Geometry check sheet. Reference: the model listing, model coordinates, mm. A direction names the side the tool comes from. Give positions to 0.01 mm unless a question says otherwise; leave off trailing zeros. Loops run counter-clockwise (first coordinate to the right, second up) from the corner with the lowest first, then second, coordinate; pieces in that order, holes last. Notation, with made-up numbers: (47, 67) -> (92, 67) arc R25 cw to (92, 93) -> close; hole circle Ø9 at (-3.75, 34.25). An arc over 180 degrees is marked (long way). Write item = value, one per line. Start each with the question number.
```python
from build123d import *

# Parameters (mm, degrees)
F0_R     = 4.35
F1_DEPTH = 15
F0_R_2   = 7
F2_DEPTH = 2
F3_D     = 5.5


with BuildPart() as f1:
    # F0 (on Top) → F1 (new body)
    with BuildSketch(Plane.XY):
        Circle(F0_R)
    extrude(amount=F1_DEPTH)

    # F0 (on Top) → F2 (join)
    with BuildSketch(Plane.XY):
        Circle(F0_R_2)
        Circle(F0_R, mode=Mode.SUBTRACT)
    extrude(amount=F2_DEPTH)

    # F3 (through all)
    with Locations(Plane(origin=(0, 0, 0), x_dir=(1, 0, 0), z_dir=(0, 0, -1))):
        with Locations((0, 0)):
            Hole(F3_D / 2)


solid = f1.part
```
1) Section check C-C (z = 6.75). Enter the section's corners in (x, y).
2) Section check D-D (x = 4). Enter the section's corners in (y, z), plus the area to 3 significant figures.
3) Draft check along X on faces 1 (the flat face through (0, -3, 0)), 2 (the cylindrical face through (6.466, -2.681, 0.986)), 3 (the cylindrical face through (0.596, 2.685, 7.605)). Enter one of: released by +X, released by -X, zero draft, split by the parting line, or undercut.
4) Section check A-A (x = 0). Enter the section's corners in (y, z), plus the area to 3 significant figures.
5) Thickness scan on line 1 (Y direction, x = 0, z = 5); line 2 (Z direction, x = -2.5, y = -4.75); line 3 (X direction, y = 0.5, z = 12). Record the ranges inside material, lowest first.
6) Tool access check on faces 4 (the flat face through (0, -3, 15)), 5 (the flat face through (0, -5, 2)). Record the directions out of +Z, -Z, +X, -X, +Y, -Y that give a thin tool (end or side, any length) a straight path to the whole face; none if there is none.
7) Depth check by flat-ended pin: pin 1 Ø1 at (x, z) = (-3.5, 5.5) entering from -Y; pin 2 Ø8 at (y, z) = (-5, 10.5) entering from -X; pin 3 Ø8 at (x, z) = (4, 13) entering from +Y. Enter the tip coordinate at first touch or a pass-through.
Check result:
q1.outline = circle Ø8.7 at (0, 0); hole circle Ø5.5 at (0, 0)
q2.outline = (-5.74, 0) -> (5.74, 0) -> (5.74, 2) -> (1.71, 2) -> (1.71, 15) -> (-1.71, 15) -> (-1.71, 2) -> (-5.74, 2) -> close
q2.area = 67.4 mm2
q3.face_1 = zero draft
q3.face_2 = split by the parting line
q3.face_3 = undercut
q4.outline = (-7, 0) -> (-2.75, 0) -> (-2.75, 15) -> (-4.35, 15) -> (-4.35, 2) -> (-7, 2) -> close; (2.75, 0) -> (7, 0) -> (7, 2) -> (4.35, 2) -> (4.35, 15) -> (2.75, 15) -> close
q4.area = 58.6 mm2
q5.line_1 = -4.35 to -2.75, 2.75 to 4.35
q5.line_2 = 0 to 2
q5.line_3 = -4.32 to -2.7, 2.7 to 4.32
q6.face_4 = +Z, +X, -X, +Y, -Y
q6.face_5 = +Z
q7.pin_1 = -3.15
q7.pin_2 = -4.23
q7.pin_3 = 4.35
